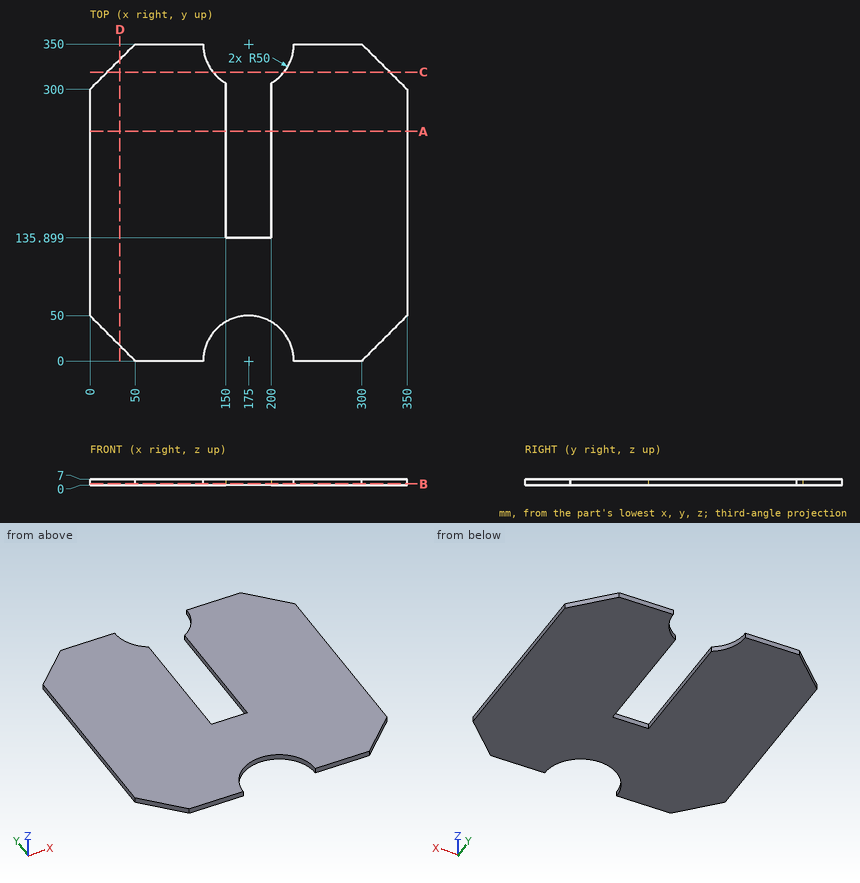
Geometry check sheet. Reference: drawing and pictorial views, mm from the part's lowest x, y, z. Give positions to 0.01 mm unless a question says otherwise; leave off trailing zeros. Order: outer loops, then holes, each group sorted by start corner. A loop starts at its lowest first (then second) coordinate and runs counter-clockwise, first axis right, second up. Notation, with made-up numbers: M 75,50.5 L 108,50.5 A29 cw 108,82.5 Z; hole C 6.25,4.25 d9. An arc over 180 degrees is marked long. Return JSON: item names as keys, results as strings. Group by question number.
1) Go/stop test with flat-tipped pins: pin 1 Ø6 at (x, y) = (94, 217.5) entering from -Z; pin 2 Ø3.5 at (x, z) = (185, 5) entering from +Y. Record where each tip stops, or that it passes through.
2) Section check D-D on x = 33. Record the cut outline in (y, z), and give its area (3 significant figures).
3) Section check A-A on y = 253.5. Record the cut outline in (x, z).
4) Scan lines: line 1 (X direction, y = 179, z = 2); line 2 (X direction, y = 39, z = 2); line 3 (Y direction, x = 317, z = 0.75). Record each from-to range of solid material in increasing order.
5) Section check B-B on z = 1.75. Record the cut outline in (x, y).
6) Section check C-C on y = 319. Record the cut outline in (x, z).
Answer block:
{
 "1": {"pin 1": "stops at z = 0", "pin 2": "stops at y = 135.9"},
 "2": {"outline": "M 17,0 L 333,0 L 333,7 L 17,7 Z", "area": "2,210 mm^2"},
 "3": {"outline": "M 0,0 L 150,0 L 150,7 L 0,7 Z; M 200,0 L 350,0 L 350,7 L 200,7 Z"},
 "4": {"line 1": "x = 0 to 150, 200 to 350", "line 2": "x = 11 to 143.71, 206.29 to 339", "line 3": "y = 17 to 333"},
 "5": {"outline": "M 0,50 L 50,0 L 125,0 A50 cw 225,0 L 300,0 L 350,50 L 350,300 L 300,350 L 225,350 A50 cw 200,306.7 L 200,135.9 L 150,135.9 L 150,306.7 A50 cw 125,350 L 50,350 L 0,300 Z"},
 "6": {"outline": "M 19,0 L 135.77,0 L 135.77,7 L 19,7 Z; M 214.23,0 L 331,0 L 331,7 L 214.23,7 Z"}
}
